```python
from build123d import *

# Parameters (mm, degrees)
SKETCH_1_R          = 3.5
EXTRUDE_1_DEPTH     = 4
SKETCH_2_R          = 2
EXTRUDE_2_DEPTH     = 20
CUT_EXTRUDE_1_DEPTH = 2
FILLET_1_R          = 0.5


with BuildPart() as part:
    # 草图1 → 凸台-拉伸1 (new body)
    with BuildSketch(Plane(origin=(0, 0, 0), x_dir=(1, 0, 0), z_dir=(0, 1, 0))):
        with Locations(Location((0, 0, 0), (0, 0, 270))):
            Circle(SKETCH_1_R)
    extrude(amount=EXTRUDE_1_DEPTH)

    # 草图2 → 凸台-拉伸2 (add)
    with BuildSketch(Plane(origin=(0, 4, 0), x_dir=(1, 0, 0), z_dir=(0, 1, 0))):
        with Locations(Location((0, 0, 0), (0, 0, 270))):
            Circle(SKETCH_2_R)
    extrude(amount=EXTRUDE_2_DEPTH)

    # 草图3 → 切除-拉伸1 (cut)
    with BuildSketch(Plane.XZ):
        Polygon((1.5, 0), (0.75, 1.299038106), (-0.75, 1.299038106), (-1.5, 0), (-0.75, -1.299038106), (0.75, -1.299038106), align=None)
    extrude(amount=-CUT_EXTRUDE_1_DEPTH, mode=Mode.SUBTRACT)

    # 圆角1
    fillet_1_edges = [part.edges().sort_by_distance(p)[0] for p in [
        (0, 0, -3.5),
        (0, 4, -3.5),
    ]]
    fillet(fillet_1_edges, radius=FILLET_1_R)


solid = part.part
```
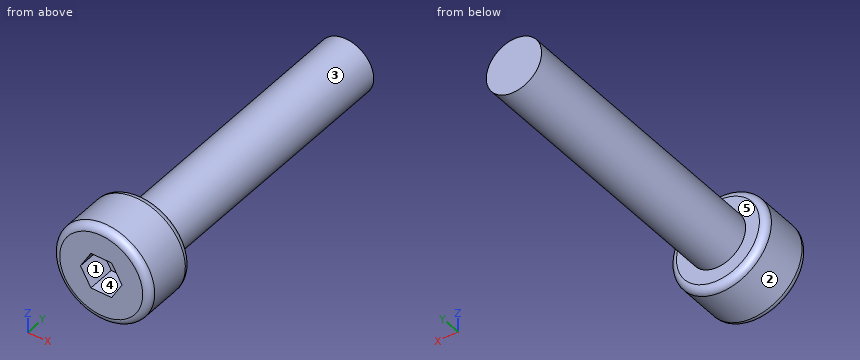
Geometry check sheet. Reference: the model listing, model coordinates, mm. Face numbers are marked on the shaded views. A direction names the side the tool comes from. Coordinates: 2 decimals unless noted, no trailing zeros. Order: outer loops, then holes, each group sorted by start corner. A loop starts at its lowest first (then second) coordinate and runs counter-clockwise, first axis right, second up. Notation, with made-up numbers: M 73.25,79.25 L 129.25,79.25 A26 ccw 129.25,114.25 Z; hole C 33,9.5 d9. An arc over 180 degrees is marked long. One line per question, with ' | ' between items. Start each with the question number.
Item 1: Gauge pin test, flat ends, axial feed: pin 1 (1.8 mm diameter, centred on x = 1.5, z = 1.5, fed in from +Y); pin 2 (2 mm diameter, centred on x = 2.5, y = 11, fed in from +Z); pin 3 (2 mm diameter, centred on y = 11.5, z = 2.5, fed in from +X); pin 4 (3 mm diameter, centred on y = 21.5, z = 2.5, fed in from +X). Record the tip position at first contact, or that the pin passes through.
Item 2: Material ranges on L1, parallel to Y at x = 0.25, z = 3; L2, parallel to X at y = 1.75, z = -1.25; L3, parallel to Z at x = 1, y = 7.5, recorded low to high. Write a range as [from, to].
Item 3: Cross-section at B-B on y = 18.25. Enter the section's corners in (x, z), then the cut area to 3 significant figures.
Item 4: Set-up check for the marked faces 1 and 2: record each of +Z, -Z, +X, -X, +Y, -Y from which the full face is reachable in a straight line by a thin tool's end or side.
Item 5: Draft check along Z on the marked faces 3, 4 and 5. Enter one of: pulls with the +Z half, pulls with the -Z half, needs draft (parallel to the pull), parting line crosses it, or undercut.
Item 6: Cross-section at A-A on x = 0. Enter the section's corners in (y, z).
Findings:
1) pin 1: stops at y = 24 | pin 2: stops at z = 1.32 | pin 3: stops at x = 1.32 | pin 4: stops at x = 1.73
2) L1: y = [0, 4] | L2: x = [-3.27, -0.78], [0.78, 3.27] | L3: z = [-1.73, 1.73]
3) outline: C 0,0 d4 | area: 12.6 mm²
4) face 1: -Y | face 2: +Y, -Y
5) face 3: parting line crosses it | face 4: undercut | face 5: needs draft
6) outline: M 0,-3 A0.5 ccw 0.5,-3.5 L 3.5,-3.5 A0.5 ccw 4,-3 L 4,-2 L 24,-2 L 24,2 L 4,2 L 4,3 A0.5 ccw 3.5,3.5 L 0.5,3.5 A0.5 ccw 0,3 L 0,1.3 L 2,1.3 L 2,-1.3 L 0,-1.3 Z
